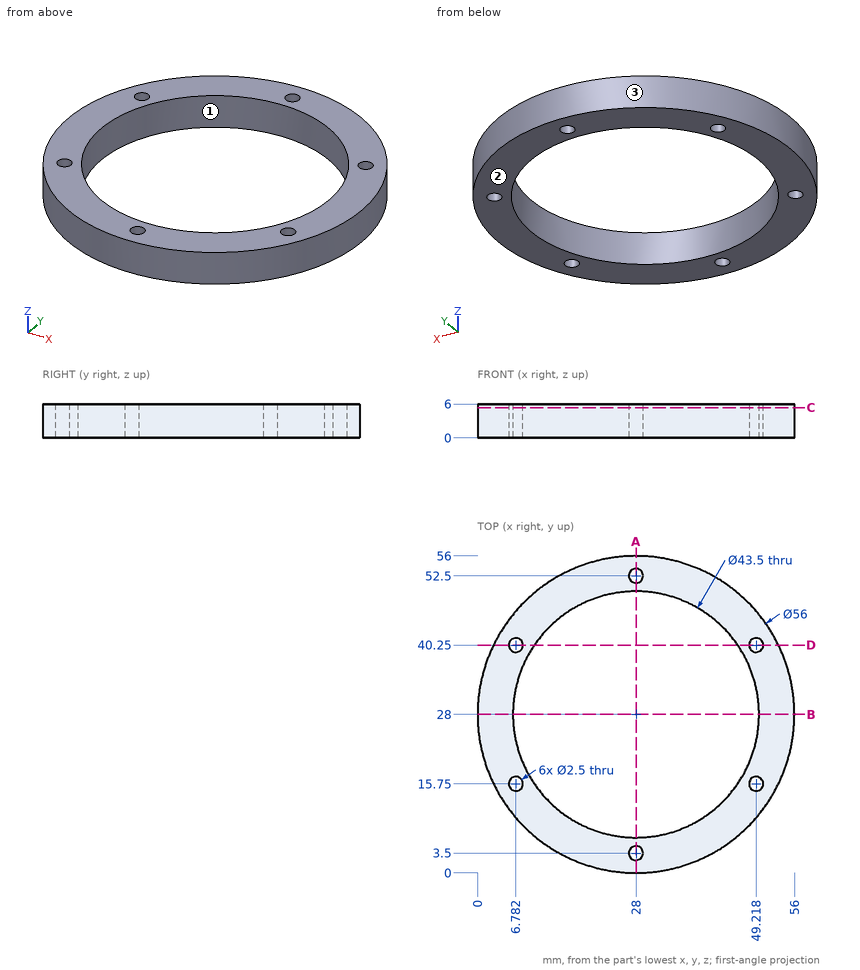
Design review of the part shown in the three views and the two pictorial views. Dimensions are in mm from the part's minimum x, y and z. Coordinates: 2 decimals unless noted, no trailing zeros. Loops run counter-clockwise (first coordinate to the right, second up) from the corner with the lowest first, then second, coordinate; pieces in that order, holes last. Notation, with made-up numbers: M -34.75,26 L -6.75,26 A23 cw -6.75,44 Z; hole C 78,53 d6. An arc over 180 degrees is marked long. Put each result on its own line as item: value. Start each with the question number.
Q1. Add section C-C (z = 5.35). Write out the cut boundary in (x, y).
Q2. Add section D-D (y = 40.25). Write out the cut boundary in (x, z).
Q3. Add section B-B (y = 28). Write out the cut boundary in (x, z), and give its area (3 significant figures).
Q4. Wall thickness on line 1 (Y direction, x = 28, z = 3.55); line 2 (X direction, y = 27.5, z = 4.85) (1 decimal); line 3 (X direction, y = 15, z = 5.4): over which ranges is each line inside the solid? List them lowest first.
Q5. Clearance check with flat-ended pins moving along their axes: pin 1 (2 mm diameter, centred on x = 28, y = 52.5, fed in from -Z); pin 2 (1 mm diameter, centred on x = 25, z = 5, fed in from -Y). State where each tip first meets the part, or that it passes through.
Q6. The part is to be moulded in two halves that separate along Y. For the marked faces 1, 2 and 3, say which applies: +Y half, -Y half, draft (parallel to the pull), parting line (faces both ways), or undercut.
Q7. Add section A-A (x = 28). Write out the cut boundary in (y, z).
Answers:
1. outline: C 28,28 d56; hole C 6.78,15.75 d2.5; hole C 6.78,40.25 d2.5; hole C 28,28 d43.5; hole C 28,3.5 d2.5; hole C 28,52.5 d2.5; hole C 49.22,15.75 d2.5; hole C 49.22,40.25 d2.5
2. outline: M 2.82,0 L 5.53,0 L 5.53,6 L 2.82,6 Z; M 8.03,0 L 10.03,0 L 10.03,6 L 8.03,6 Z; M 45.97,0 L 47.97,0 L 47.97,6 L 45.97,6 Z; M 50.47,0 L 53.18,0 L 53.18,6 L 50.47,6 Z
3. outline: M 0,0 L 6.25,0 L 6.25,6 L 0,6 Z; M 49.75,0 L 56,0 L 56,6 L 49.75,6 Z
3. area: 75.0 mm^2
4. line 1: y = 0 to 2.25, 4.75 to 6.25, 49.75 to 51.25, 53.75 to 56
4. line 2: x = 0 to 6.3, 49.7 to 56
4. line 3: x = 3.2 to 5.78, 7.78 to 10.56, 45.44 to 48.22, 50.22 to 52.8
5. pin 1: passes through
5. pin 2: stops at y = 0.11
6. face 1: undercut
6. face 2: draft
6. face 3: parting line
7. outline: M 0,0 L 2.25,0 L 2.25,6 L 0,6 Z; M 4.75,0 L 6.25,0 L 6.25,6 L 4.75,6 Z; M 49.75,0 L 51.25,0 L 51.25,6 L 49.75,6 Z; M 53.75,0 L 56,0 L 56,6 L 53.75,6 Z
